Could you check a few things on this drawing? It's one solid part, dimensions in mm from its lowest x, y, z. A direction names the side the tool comes from. Give positions to 0.01 mm unless a question says otherwise; leave off trailing zeros. Order: outer loops, then holes, each group sorted by start corner. A loop starts at its lowest first (then second) coordinate and runs counter-clockwise, first axis right, second up. Notation, with made-up numbers: (50.25, 27.5) - (74.25, 27.5) arc R14 cw to (74.25, 51.5) - close; hole circle Ø9 at (-37, -12.75). An arc over 180 degrees is marked (long way). One line per question, with ' | ' between items. Start each with the question number.
1. For P1, Ø18.5, axis at x = 50, y = 36.5, coming from the +Z side (1 decimal), with a flat end and sliding along its axis, tell me the tip position at first contact or that it passes through.
2. Imagine slicing it at B-B (y = 37.5). Please give me the cut outline in (x, z) (1 decimal), and give its area (3 significant figures).
3. I need wall thicknesses on probe 1 along X at (y, z) = (51, 15.5); probe 2 along Z at (x, y) = (70.5, 16.5) (1 decimal); probe 3 along Y at (x, z) = (56, 9) (1 decimal). Which ranges of each line are inside material? Lowest first, please. Write a range as from..to.
4. Imagine slicing it at A-A (y = 52.5). Please give me the cut outline in (x, z) (1 decimal), and give its area (3 significant figures).
5. If we mould it in two halves opening along Y, with no side actions, what happens to the marked faces 3, 4 and 5? For each: released by +Y, released by -Y, zero draft, split by the parting line, or undercut.
6. Imagine slicing it at C-C (z = 45). Please give me the cut outline in (x, y) (1 decimal), and give its area (4 significant figures).
7. Imagine slicing it at D-D (x = 39.5). Please give me the cut outline in (y, z) (1 decimal).
8. Which directions (+Z, -Z, +X, -X, +Y, -Y) give clear straight access to the entire face, cutting with the end or side of a thin tool? Please do the marked faces 1 and 2.
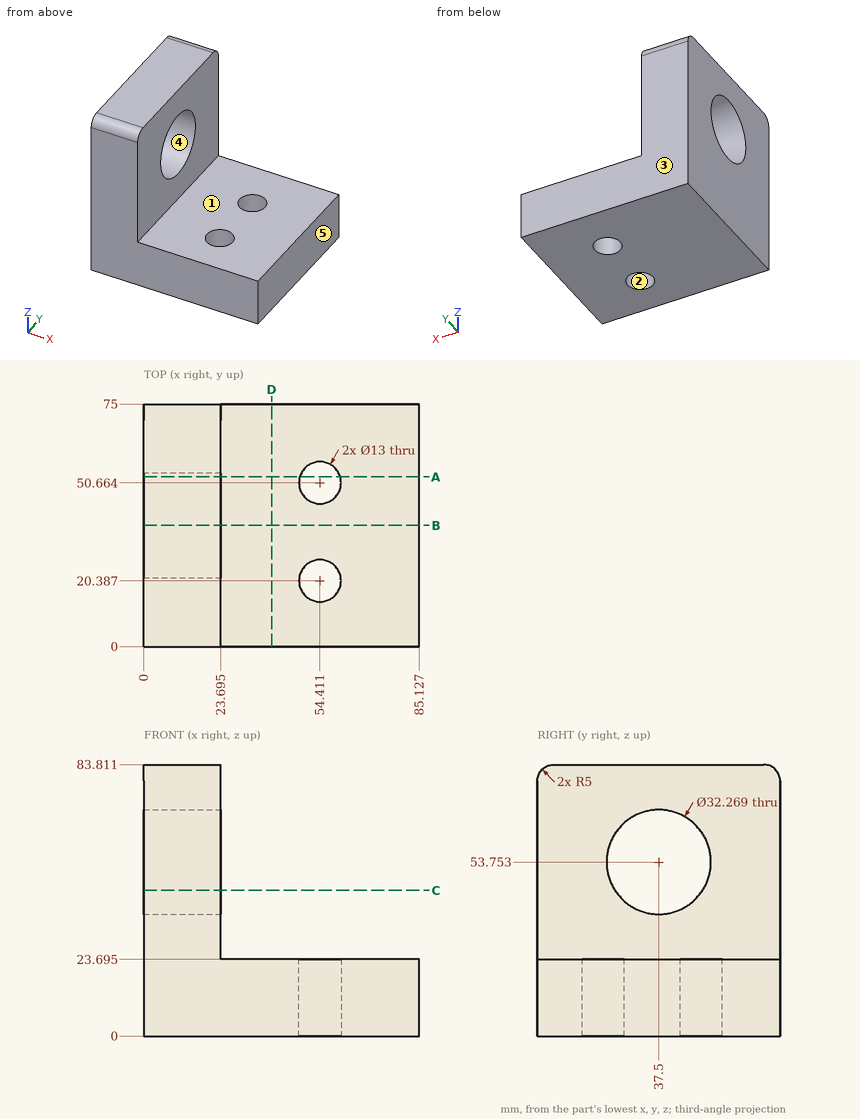
Results found:
1) P1: stops at z = 23.7
2) outline: (0, 0) - (85.1, 0) - (85.1, 23.7) - (23.7, 23.7) - (23.7, 37.6) - (0, 37.6) - close; (0, 69.9) - (23.7, 69.9) - (23.7, 83.8) - (0, 83.8) - close | area: 2,680 mm2
3) probe 1: x = 0..47.92, 60.9..85.13 | probe 2: z = 0..23.7 | probe 3: y = 0..14.1, 26.7..44.4, 57..75
4) outline: (0, 0) - (48.2, 0) - (48.2, 23.7) - (23.7, 23.7) - (23.7, 47.8) - (0, 47.8) - close; (0, 59.7) - (23.7, 59.7) - (23.7, 83.8) - (0, 83.8) - close; (60.6, 0) - (85.1, 0) - (85.1, 23.7) - (60.6, 23.7) - close | area: 2,860 mm2
5) face 3: released by +Y | face 4: undercut | face 5: zero draft
6) outline: (0, 0) - (23.7, 0) - (23.7, 23.9) - (0, 23.9) - close; (0, 51.1) - (23.7, 51.1) - (23.7, 75) - (0, 75) - close | area: 1,135 mm2
7) outline: (0, 0) - (75, 0) - (75, 23.7) - (0, 23.7) - close
8) face 1: +Z, +X, +Y, -Y | face 2: +Z, -Z
